The listing builds one solid part. Answer for the finished solid, in the listing's coordinates (mm). A direction names the side the tool comes from. Coordinates: 2 decimals unless noted, no trailing zeros. Write each loop counter-clockwise with the first axis right and the second up, starting at its lowest first coordinate (ties: lowest second). Pieces come first, ordered by that corner, then holes.
(1) For a pull along Z with two mould halves and no side action, classify faces 4 (the conical face through (0.095, 0.136, -0.043)), 5 (the flat face through (-2.18, -0.98, 1.72)), 6 (the flat face through (12.7, 0, 0)), 7 (the cylindrical face through (5.93, -0.69, 3.1)) as +Z half, -Z half, draft (parallel to the pull), parting line (faces both ways), or undercut.
(2) Given P1, Ø3, axis at x = 4, z = 3, coming from the +Y side; P2, Ø2.5, axis at x = -2.5, z = -0.5, coming from the -Y side; P3, Ø1, axis at y = 3, z = -2.5, coming from the -X side, each flat-ended and moving along its own axis, determine where each tip first touches the part or whether it passes through.
(3) Straight lines are drawn through the part: line 1 (Z direction, x = -0.5, y = -5); line 2 (X direction, y = 4.75, z = -1); line 3 (X direction, y = -0.25, z = -4). For each, find the intervals that lie inside material, in ascending order.
(4) Which of the six approach directions +Z, -Z, +X, -X, +Y, -Y give full straight-line access (tool end or side, diameter ignored) to faces 1 (the flat face through (-2, 1.981, 0)), 2 (the conical face through (0, 3.3, -1)), 3 (the flat face through (-3.353, 1, 2))?
(5) The part is cut by section A-A on x = 5.25. Determine the outline of the cut face in (y, z) (3 decimals).
Autodesk Inventor part; units mm, degrees
ref_plane "Work Plane1" through (29, 0, 0) normal (0, -1, 0) x (1, 0, 0)
ref_plane "YZ Plane" through (0, 0, 0) normal (1, 0, 0) x (0, 1, 0)
ref_plane "XZ Plane" through (0, 0, 0) normal (0, 1, 0) x (-1, 0, 0)
sketch "Sketch1" plane through (0, 0, 0) normal (0, 0, 1) x (1, 0, 0)
  line L0 (0.1778, 0) -> (12.7, 0)
  line L1 (12.7, 0) -> (12.7, 3.175)
  line L2 (12.7, 3.175) -> (2.5402, 3.175)
  line L3 (2.5402, 3.175) -> (0.0001, 3.175)
  line L4 (0.0001, 3.175) -> (0, 3.175)
  line L5 (0, 3.175) -> (0, 5.5499)
  line L6 (0, 5.5499) -> (-3.3528, 5.5499)
  line L7 (-3.3528, 5.5499) -> (-3.3528, 2.2877)
  line L8 (-3.3528, 2.2877) -> (-1.143, 2.2877)
  line L9 (-1.143, 2.2877) -> (0.1778, 0)
  line L10 (-6.5634, 0) -> (15.9106, 0)
  line L11 (0, -1.11) -> (0, 6.6599)
  line L12 (2.5402, 3.175) -> (0, 3.175) construction
  dimension "d1" = 10.1598
  dimension "d2" = 2.5401
  dimension "d3" = 3.3528
  dimension "d4" = 2.2098
  dimension "d5" = 60
  dimension "d6" = 6.35
  dimension "d7" = 6.35
  dimension "d8" = 4.5754
  dimension "d9" = 11.0998
  dimension "d26" = 12.7
revolve "Body" add sketch "Sketch1" angle 360 about axis through (0.1778, 0, 0) along (1, 0, 0) contours L9 L11 L3 L2 L1 L0 | L9 L8 L7 L6 L5 L11
sketch "Sketch2" plane through (-3.3528, 0, 0) normal (-1, 0, 0) x (0, 0, 1)
  circle A0 centre (0, 0) radius 2.2877
  line L0 (0, -7.7699) -> (0, 7.7699)
  line L1 (-7.7699, 0) -> (7.7699, 0)
  line L2 (2.2877, 0) -> (1.1438, -1.9812)
  line L3 (1.1438, -1.9812) -> (-1.1438, -1.9812)
  line L4 (-1.1438, -1.9812) -> (-2.2877, 0)
  line L5 (-2.2877, 0) -> (-1.1438, 1.9812)
  line L6 (-1.1438, 1.9812) -> (1.1438, 1.9812)
  line L7 (1.1438, 1.9812) -> (2.2877, 0)
  point P0 (0, 0)
extrude "Slot" add sketch "Sketch2" against normal up to next contours L7 A0 | A0 L2 | L6 L0 A0 | A0 L0 L3 | L0 L6 A0 | A0 L3 L0 | L4 A0 | A0 L5
fillet "Fillet1" radius 2.9718 1 edges at (-3.3528, -5.5499, 0)
thread "Thread"
chamfer "Chamfer1" distance 0.779 distance2 0.779 1 edges at (12.7, -3.175, 0) measured on face at (12.7, -1.2091, -0.9896)
ref_plane "Work Plane1" through (29, 0, 0) normal (0, -1, 0) x (1, 0, 0)
fillet "Fillet2" radius 0.1 1 edges at (0.0001, -3.175, 0)
equation "\"d1\" = GEL"
equation "\"d3\" = KOH"
equation "\"d4\" = INTI"
equation "\"d6\" = GD"
equation "\"d7\" = BDM"
equation "\"d8\" = 1.1547 * SW"
equation "\"d9\" = KOD"
equation "\"d26\" = NLG"
equation "\"d30\" = R"
equation "\"d17\" = RR"
equation "\"d13\" = GEL"
equation "\"d15\" = -0.5 * SPD + 0.5 * GD"
equation "\"d16\" = GUL"
equation "\"GD\" = NND"
equation "\"NLG\" = 12.7"
equation "\"GEL\" = 10.1598"
equation "\"KOD\" = 11.0998"
equation "\"KOH\" = 3.3528"
equation "\"INTI\" = 2.2098"
equation "\"GAL\" = 2.54"
equation "\"GUL\" = 0.77902"
equation "\"BDM\" = NND"
equation "\"SW\" = 3.9624"
equation "\"RR\" = 2.9718"
equation "\"SPD\" = 4.79196"
equation "\"R\" = 0.1"
equation "\"TOA\" = 30deg"
equation "\"GD1\" = SPD"
equation "\"THREADDIA\" = 6.35"
equation "\"KOH1\" = 0.7874"
equation "\"NND\" = 6.35"
equation "\"E0\" = 4.57657"
properties part number "am-1039" material "Steel, Mild"
Model answer:
1. face 4: undercut
1. face 5: undercut
1. face 6: draft
1. face 7: parting line
2. P1: stops at y = 2.8
2. P2: stops at y = -5.41
2. P3: stops at x = -3.24
3. line 1: z = -2.4 to 2.4
3. line 2: x = -2.29 to 0
3. line 3: x = -2.99 to 0
4. face 1: -X
4. face 2: +X
4. face 3: +Z, -Z, -X, +Y, -Y
5. outline: circle Ø6.35 at (0, 0)
